Source: CAD feature listing. Evaluate the final solid. Frame: model axes, mm. A direction names the side the tool comes from. Give positions to 0.01 mm unless a question says otherwise; leave off trailing zeros. Loops run counter-clockwise (first coordinate to the right, second up) from the corner with the lowest first, then second, coordinate; pieces in that order, holes last. Notation, with made-up numbers: (69.5, -39) - (77.5, -39) arc R8 cw to (77.5, -33) - close; hole circle Ø7 at (-25, -5). An arc over 180 degrees is marked (long way). Write each question's results on one line, items separated by ' | '. Start each with the question number.
(1) Reachability of faces 1 (the flat face through (-23.539, 9, 2)), 2 (the flat face through (-22, 4.301, 2)), 3 (the flat face through (-34, 52, 19)), 4 (the flat face through (-37.855, 51.041, 16.28)), 5 (the flat face through (-34, 50.301, 12)) from +Z, -Z, +X, -X, +Y, -Y: full face, straight path, thin tool, end or side. Return the list, or none.
(2) Cut plane C-C on z = 7.75. Return the cut outline in (x, y), then the cut area to 3 significant figures.
(3) Pull-direction query (Z, two-part tool) for faces 6 (the flat face through (-25.355, 51.041, 16.28)), 7 (the flat face through (-50.539, 36, 3)), 8 (the cylindrical face through (-18.11, 52.33, 18.4)); classes: pulls with the +Z half, pulls with the -Z half, needs draft (parallel to the pull), parting line crosses it, or undercut.
(4) Contact query for flat-ended pins moving along their axis: pin 1 (16.5 mm diameter, centred on x = -41.5, y = 18.5, fed in from +Z); pin 2 (3 mm diameter, centred on x = -33.5, z = 1.5, fed in from -Y); pin 3 (10 mm diameter, centred on x = -42, y = 44, fed in from +Z). Output: stop coordinate, or through.
(5) Material intervals for line 1 along X through (y, z) = (52.8, 15); line 2 along Y through (x, z) = (-22.5, 1.75); line 3 along Y through (x, z) = (-23.5, 15.25), sorted ascending. Write a range as [from, to].
(6) Cut plane A-A on y = 11.5. Return the cut outline in (x, z).
(7) Cut plane D-D on x = -21. Return the cut outline in (y, z), then the cut area to 3 significant figures.
(8) Cut plane B-B on x = -34.5. Return the cut outline in (y, z).
from build123d import *

# Parameters (mm, degrees)
F0_R     = 0.8
F1_DEPTH = 4
F2_W     = 33
F2_H     = 4
F3_DEPTH = 15
F4_R     = 1.6
F5_DEPTH = 25
F6_R     = 1.6
F7_DEPTH = 1.5
F8_R     = 2


with BuildPart() as f1:
    # F0 (on Top) → F1 (new body)
    with BuildSketch(Plane.XY):
        Polygon((-23.5390763283, 54.3011978269), (-44.5390763283, 54.3011978269), (-50.5390763283, 54.3011978269), (-50.5390763283, 4.3011978269), (-44.5390763283, 4.3011978269), (-44.5390763283, 13.3011978269), (-23.5390763283, 13.3011978269), (-23.5390763283, 4.3011978269), (-17.5390763283, 4.3011978269), (-17.5390763283, 54.3011978269), align=None)
        with Locations((-45.5390763283, 8.8011978269)):
            Circle(F0_R, mode=Mode.SUBTRACT)
        with Locations((-22.5390763283, 8.8011978269)):
            Circle(F0_R, mode=Mode.SUBTRACT)
    extrude(amount=F1_DEPTH)

    # F2 (on face) → F3 (join)
    with BuildSketch(Plane.XY.offset(4)):
        with Locations((-34.0390763283, 52.3011978269)):
            Rectangle(F2_W, F2_H)
    extrude(amount=F3_DEPTH)

    # F4 (on face) → F5 (cut)
    with BuildSketch(Plane(origin=(0, 54.3011978269, 0), x_dir=(-1, 0, 0), z_dir=(0, 1, 0))):
        with Locations((40.2890763283, 15)):
            Circle(F4_R)
        with Locations((27.7890763283, 15)):
            Circle(F4_R)
    extrude(amount=-F5_DEPTH, mode=Mode.SUBTRACT)

    # F6 (on face) → F7 (cut)
    with BuildSketch(Plane.XZ.offset(-50.3011978269)):
        Polygon((-38.7884142354, 12.2015456737), (-37.1152127439, 14.9003843318), (-38.6158748368, 17.6988386581), (-41.7897384212, 17.7984543263), (-43.4629399126, 15.0996156682), (-41.9622778197, 12.3011613419), align=None)
        with Locations((-40.2890763283, 15)):
            Circle(F6_R, mode=Mode.SUBTRACT)
        Polygon((-26.2884142354, 12.2015456737), (-24.6152127439, 14.9003843318), (-26.1158748368, 17.6988386581), (-29.2897384212, 17.7984543263), (-30.9629399126, 15.0996156682), (-29.4622778197, 12.3011613419), align=None)
        with Locations((-27.7890763283, 15)):
            Circle(F6_R, mode=Mode.SUBTRACT)
    extrude(amount=-F7_DEPTH, mode=Mode.SUBTRACT)

    # F8
    f8_edges = [f1.edges().sort_by_distance(p)[0] for p in [
        (-50.539076, 4.301198, 2),
        (-17.539076, 4.301198, 2),
        (-17.539076, 52.301198, 19),
        (-50.539076, 52.301198, 19),
        (-34.039076, 50.301198, 4),
    ]]
    fillet(f8_edges, radius=F8_R)


solid = f1.part
Ans:
1) face 1: +Z, -Z, -Y | face 2: +Z, -Z, +X, -X, -Y | face 3: +Z, +X, -X, +Y, -Y | face 4: -Y | face 5: +Z, +X, -X, -Y
2) outline: (-50.54, 50.3) - (-17.54, 50.3) - (-17.54, 54.3) - (-50.54, 54.3) - close | area: 132 mm^2
3) face 6: undercut | face 7: needs draft | face 8: pulls with the +Z half
4) pin 1: z = 4 | pin 2: y = 13.3 | pin 3: z = 4.13
5) line 1: [-50.54, -41.89], [-38.69, -29.39], [-26.19, -17.54] | line 2: [4.3, 8], [9.6, 54.3] | line 3: [50.3, 54.3]
6) outline: (-50.54, 0) - (-44.54, 0) - (-44.54, 4) - (-50.54, 4) - close; (-23.54, 0) - (-17.54, 0) - (-17.54, 4) - (-23.54, 4) - close
7) outline: (4.3, 0) - (54.3, 0) - (54.3, 19) - (50.3, 19) - (50.3, 6) arc R2 cw to (48.3, 4) - (4.3, 4) - close | area: 261 mm^2
8) outline: (13.3, 0) - (54.3, 0) - (54.3, 19) - (50.3, 19) - (50.3, 6) arc R2 cw to (48.3, 4) - (13.3, 4) - close
